from build123d import *

# Parameters (mm, degrees)
F0_R     = 28.722262
F1_DEPTH = 203.2
F2_W     = 14.590031
F2_H     = 7.466263
F3_DEPTH = 101.6
F5_DEPTH = 101.6
F6_R     = 11.300877
F7_DEPTH = 76.2


with BuildPart() as f1:
    # F0 (on Top) → F1 (new body)
    with BuildSketch(Plane.XY):
        Circle(F0_R)
    extrude(amount=F1_DEPTH)

    # F2 (on face) → F3 (join)
    with BuildSketch(Plane.XY.offset(203.2)):
        with Locations((7.295015, 3.733131)):
            Rectangle(F2_W, F2_H)
    extrude(amount=F3_DEPTH)

    # F4 (on face) → F5 (join)
    with BuildSketch(Plane.XZ):
        Polygon((38.268968, 226.788725), (49.995155, 260.900924), (26.316217, 288.112199), (-9.088907, 281.211275), (-20.815094, 247.099076), (2.863844, 219.887801), align=None)
    extrude(amount=F5_DEPTH)

    # F6 (on face) → F7 (cut)
    with BuildSketch(Plane.XZ.offset(101.6)):
        with Locations((13.679512, 253.768682)):
            Circle(F6_R)
    extrude(amount=-F7_DEPTH, mode=Mode.SUBTRACT)


solid = f1.part
Work out the finished part from the listing and answer in its coordinate system (mm). A direction names the side the tool comes from. Give positions to 0.01 mm unless a question says otherwise; leave off trailing zeros. Order: outer loops, then holes, each group sorted by start corner. A loop starts at its lowest first (then second) coordinate and runs counter-clockwise, first axis right, second up. Notation, with made-up numbers: (14.25, -39) -> (42.25, -39) arc R20 cw to (42.25, -26) -> close; hole circle Ø3 at (-29, -18). An arc over 180 degrees is marked (long way). Answer as a JSON object with one key per item and string values. Group by question number.
1. A tool of negligible diameter and unlimited length cuts with its end or side. For faces 1 (the flat face through (7, 0, 294)), 2 (the flat face through (-8, 0, 253)), 3 (the flat face through (14, -25.4, 254)), 4 (the flat face through (28, 0, 256)), 5 (the flat face through (20.32, -50.09, 223.29)), from which of +Z, -Z, +X, -X, +Y, -Y can it reach the whole face along a straight path? Write none if from no direction.
2. Flat-ended cylindrical pins translate along their axes: pin 1 Ø23 at (x, z) = (-12.5, 254) entering from +Y; pin 2 Ø5 at (x, z) = (5.5, 197.5) entering from -Y; pin 3 Ø5 at (x, z) = (20, 176) entering from +Y. Find the tip coordinate at first contact, or state that the pin passes through.
3. Section C-C on z = 72 is taken. Determine the outline of the cut face in (x, y), plus the area to 3 significant figures.
4. The mould has two halves that part along Z. Classify faces 6 (the flat face through (-9.14, -50.09, 233.68)), 7 (the flat face through (-14.87, -50.09, 264.39)), 8 (the flat face through (7, 7.466, 253)): released by +Z, released by -Z, zero draft, split by the parting line, or undercut.
5. Section A-A on y = -5.5 is taken. Determine the outline of the cut face in (x, z), plus the area to 3 significant figures.
6. Consider line 1 along Y through (x, z) = (-3, 231.5); line 2 along Z through (x, y) = (9.5, -91); line 3 along Z through (x, y) = (6, -33). Determine where each line is inside the solid, lowest interval first. Write a range as [from, to].
7. Section D-D on y = -32 is taken. Determine the outline of the cut face in (x, z), plus the area to 3 significant figures.
8. Section B-B on x = -4.5 is taken. Determine the outline of the cut face in (y, z).
Result sheet:
{
 "1": {"face 1": "+Z, -X, -Y", "face 2": "+Z, -X, +Y", "face 3": "-Y", "face 4": "+Z, +X, +Y", "face 5": "+X, -Y"},
 "2": {"pin 1": "stops at y = 0", "pin 2": "stops at y = -28.57", "pin 3": "stops at y = 22.78"},
 "3": {"outline": "circle Ø57.44 at (0, 0)", "area": "2,590 mm^2"},
 "4": {"face 6": "undercut", "face 7": "released by +Z", "face 8": "zero draft"},
 "5": {"outline": "(-28.19, 0) -> (28.19, 0) -> (28.19, 203.2) -> (-28.19, 203.2) -> close; (-20.82, 247.1) -> (2.86, 219.89) -> (38.27, 226.79) -> (50, 260.9) -> (26.32, 288.11) -> (-9.09, 281.21) -> close", "area": "14,800 mm^2"},
 "6": {"line 1": "y = [-101.6, 0]", "line 2": "z = [221.18, 243.27], [264.27, 284.83]", "line 3": "z = [220.5, 245.48], [262.06, 284.15]"},
 "7": {"outline": "(-20.82, 247.1) -> (2.86, 219.89) -> (38.27, 226.79) -> (50, 260.9) -> (26.32, 288.11) -> (-9.09, 281.21) -> close; hole circle Ø22.6 at (13.68, 253.77)", "area": "2,980 mm^2"},
 "8": {"outline": "(-101.6, 228.35) -> (0, 228.35) -> (0, 282.11) -> (-101.6, 282.11) -> close; (-28.37, 0) -> (28.37, 0) -> (28.37, 203.2) -> (-28.37, 203.2) -> close"}
}
